Input: part model. Units: mm. Frame: model coordinates. A direction names the side the tool comes from. Round coordinates to 2 decimals unless told otherwise and drop trailing zeros. Loops run counter-clockwise (first coordinate to the right, second up) from the corner with the lowest first, then second, coordinate; pieces in that order, holes last. Notation, with made-up numbers: (-6, 37.25) -> (13, 37.25) arc R22 ccw to (13, 52.25) -> close; hole circle Ø10 at (35, 29.5). An arc over 180 degrees is marked (long way). Answer in a Markdown table with one row per item. Add a question column.
Q1. Reachability of faces 4 (the face through (-3, -16, 15)), 5 (the face through (-14, -30, 7)) from +Z, -Z, +X, -X, +Y, -Y: full face, straight path, thin tool, end or side. Return the list, or none.
Q2. Section A-A, the plane y = 2. Output: boundary loops of the cut face in (x, z).
Q3. Mould query, pull axis Y, two halves, no side actions, for faces 1 (the face through (0.16, 7.5, 7.4)), 2 (the face through (-0.54, -2.44, 7.4)), 3 (the face through (-3, -16, 0)). Classes: pulls with the +Y half, pulls with the -Y half, needs draft (parallel to the pull), parting line crosses it, or undercut.
Q4. Pin query (flat end, axial travel): pin 1 (4 mm diameter, centred on x = 0, y = 0, fed in from -Z); pin 2 (2 mm diameter, centred on x = -2, z = 11, fed in from -Y); pin 3 (1.2 mm diameter, centred on x = -14.5, z = 9.5, fed in from +Y). Return the tip coordinate at first contact, or that it passes through.
Q5. Ray query, L1, parallel to X at y = -4, z = 1.5; L2, parallel to Y at x = 0, z = 3; L3, parallel to Y at x = 1.5, z = 13. Return the intervals inside material, ascending. Write a range as from..to.
```python
from build123d import *

# Parameters (mm, degrees)
BOSS_EXTRUDE1_DEPTH     = 15
CUT_EXTRUDE1_DEPTH      = 46.276925845
CUT_EXTRUDE1_DEPTH_BACK = 46.276925845
SKETCH2_R               = 2.5


with BuildPart() as part:
    # Sketch1 → Boss-Extrude1 (new body)
    with BuildSketch(Plane.XY):
        with BuildLine():
            Line((-15, -40), (-13.5, -40))
            add(Edge.make_bspline(
                [(7.5, 0), (9.663811458, -23.774808376), (-13.5, -40)],
                knots=[0, 0, 0, 1, 1, 1], degree=2))
            ThreePointArc((7.5, 0), (0, 7.5), (-7.5, 0))
            add(Edge.make_bspline(
                [(-7.5, 0), (-6.464333995, -15.538187235), (-13.5, -30)],
                knots=[0, 0, 0, 1, 1, 1], degree=2))
            Line((-13.5, -30), (-15, -30))
            Line((-15, -30), (-15, -40))
        make_face()
    extrude(amount=BOSS_EXTRUDE1_DEPTH)

    # Sketch2 → Cut-Extrude1 (cut, two sides: drawn at the far end of the back side and taken through both)
    with BuildSketch(Plane.XY.offset(15).offset(-CUT_EXTRUDE1_DEPTH_BACK)):
        Circle(SKETCH2_R)
    extrude(amount=CUT_EXTRUDE1_DEPTH + CUT_EXTRUDE1_DEPTH_BACK, mode=Mode.SUBTRACT)


solid = part.part
```
Answer block:
| question | item | result |
|---|---|---|
| 1 | face 4 | +Z, +X, -X, +Y, -Y |
| 1 | face 5 | +Z, -Z, -X, +Y |
| 2 | outline | (-7.23, 0) -> (-1.5, 0) -> (-1.5, 15) -> (-7.23, 15) -> close; (1.5, 0) -> (7.23, 0) -> (7.23, 15) -> (1.5, 15) -> close |
| 3 | face 1 | pulls with the +Y half |
| 3 | face 2 | undercut |
| 3 | face 3 | needs draft |
| 4 | pin 1 | through |
| 4 | pin 2 | y = -30.87 |
| 4 | pin 3 | y = -30 |
| 5 | L1 | -7.37..7.68 |
| 5 | L2 | -27.2..-2.5, 2.5..7.5 |
| 5 | L3 | -25.02..-2, 2..7.35 |
